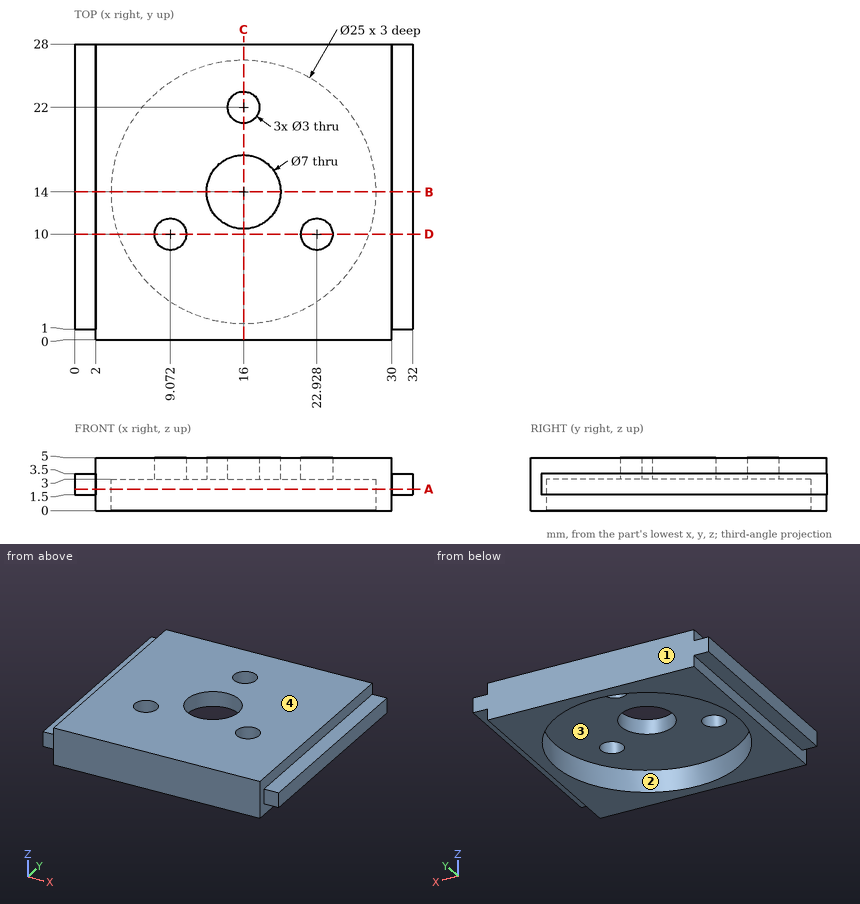
Geometry check sheet. Reference: drawing and pictorial views, mm from the part's lowest x, y, z. A direction names the side the tool comes from. Round coordinates to 2 decimals unless told otherwise and drop trailing zeros. Write each loop counter-clockwise with the first axis right and the second up, starting at its lowest first coordinate (ties: lowest second). Pieces come first, ordered by that corner, then holes.
1. Section check C-C on x = 16. Enter the section's corners in (y, z).
2. Gauge pin test, flat ends, axial feed: P1, Ø0.6, axis at x = 31, z = 2.5, coming from the -Y side; P2, Ø0.6, axis at x = 30.5, y = 13, coming from the -Z side; P3, Ø12.5, axis at x = 13.5, y = 11, coming from the -Z side. Record the tip position at first contact, or that the pin passes through.
3. Draft check along X on the marked faces 1 and 2. Enter one of: +X half, -X half, draft (parallel to the pull), parting line (faces both ways), or undercut.
4. Access from +Z, -Z, +X, -X, +Y, -Y to the whole of each face (thin tool, end or side, straight path). Record for the marked faces 3 and 4.
5. Section check B-B on y = 14. Enter the section's corners in (x, z).
6. Section check D-D on y = 10. Enter the section's corners in (x, z).
7. Scan lines: L1, parallel to Y at x = 16, z = 3.6; L2, parallel to Y at x = 23, z = 4.3; L3, parallel to Y at x = 16.5, z = 4.5. Record each from-to range of solid material in increasing order.
8. Section check A-A on z = 2.05. Enter the section's corners in (x, y).
Answer:
1. outline: (0, 0) - (1.5, 0) - (1.5, 3) - (10.5, 3) - (10.5, 5) - (0, 5) - close; (17.5, 3) - (20.5, 3) - (20.5, 5) - (17.5, 5) - close; (23.5, 3) - (26.5, 3) - (26.5, 0) - (28, 0) - (28, 5) - (23.5, 5) - close
2. P1: stops at y = 1
2. P2: stops at z = 1.5
2. P3: stops at z = 3
3. face 1: draft
3. face 2: undercut
4. face 3: -Z
4. face 4: +Z, +X, -X, +Y, -Y
5. outline: (0, 1.5) - (2, 1.5) - (2, 0) - (3.5, 0) - (3.5, 3) - (12.5, 3) - (12.5, 5) - (2, 5) - (2, 3.5) - (0, 3.5) - close; (19.5, 3) - (28.5, 3) - (28.5, 0) - (30, 0) - (30, 1.5) - (32, 1.5) - (32, 3.5) - (30, 3.5) - (30, 5) - (19.5, 5) - close
6. outline: (0, 1.5) - (2, 1.5) - (2, 0) - (4.16, 0) - (4.16, 3) - (7.57, 3) - (7.57, 5) - (2, 5) - (2, 3.5) - (0, 3.5) - close; (10.57, 3) - (21.43, 3) - (21.43, 5) - (10.57, 5) - close; (24.43, 3) - (27.84, 3) - (27.84, 0) - (30, 0) - (30, 1.5) - (32, 1.5) - (32, 3.5) - (30, 3.5) - (30, 5) - (24.43, 5) - close
7. L1: y = 0 to 10.5, 17.5 to 20.5, 23.5 to 28
7. L2: y = 0 to 8.5, 11.5 to 28
7. L3: y = 0 to 10.54, 17.46 to 20.59, 23.41 to 28
8. outline: (0, 1) - (2, 1) - (2, 0) - (30, 0) - (30, 1) - (32, 1) - (32, 28) - (0, 28) - close; hole circle Ø25 at (16, 14)
